Source: CAD feature listing. Evaluate the final solid. Frame: model axes, mm. A direction names the side the tool comes from. Give positions to 0.01 mm unless a question says otherwise; leave off trailing zeros. Loops run counter-clockwise (first coordinate to the right, second up) from the corner with the lowest first, then second, coordinate; pieces in that order, holes last.
from build123d import *

# Parameters (mm, degrees)
BOSS_EXTRUDE1_DEPTH = 25
SKETCH2_R           = 3
CUT_EXTRUDE1_DEPTH  = 11


with BuildPart() as part:
    # Sketch1 → Boss-Extrude1 (new, symmetric)
    with BuildSketch(Plane.XY):
        with BuildLine():
            Line((-24, 23), (24, 23))
            Line((24, 23), (24, -16))
            Line((24, -16), (9.237604307, -16))
            Line((9.237604307, -16), (5, -8.660254038))
            ThreePointArc((5, -8.660254038), (0, 10), (-5, -8.660254038))
            Line((-5, -8.660254038), (-9.237604307, -16))
            Line((-9.237604307, -16), (-24, -16))
            Line((-24, -16), (-24, 23))
        make_face()
    extrude(amount=BOSS_EXTRUDE1_DEPTH, both=True)

    # Sketch2 → Cut-Extrude1 (cut)
    with BuildSketch(Plane(origin=(0, 23, 0), x_dir=(1, 0, 0), z_dir=(0, 1, 0))):
        with Locations(Location((-17.5, 17.5, 0), (0, 0, 270))):
            Circle(SKETCH2_R)
        with Locations(Location((17.5, 17.5, 0), (0, 0, 270))):
            Circle(SKETCH2_R)
        with Locations(Location((17.5, -17.5, 0), (0, 0, 270))):
            Circle(SKETCH2_R)
        with Locations(Location((-17.5, -17.5, 0), (0, 0, 270))):
            Circle(SKETCH2_R)
    extrude(amount=-CUT_EXTRUDE1_DEPTH, mode=Mode.SUBTRACT)


solid = part.part
1) Pull-direction query (X, two-part tool) for faces 4 (the flat face through (-24, 3, 0)), 5 (the flat face through (0, 12, -25)), 6 (the flat face through (-17, 12, -18)); classes: released by +X, released by -X, zero draft, split by the parting line, or undercut.
Checks:
face 4: released by -X
face 5: zero draft
face 6: undercut
2) Contact query for a flat-ended pin moving along its axis: P1, Ø1.8, axis at x = 16.5, z = -18, coming from the +Y side. Output: stop coordinate, or through.
Checks:
P1: stops at y = 12
3) Ray query, probe 1 along X at (y, z) = (14.75, -17.5); probe 2 along X at (y, z) = (0, -12); probe 3 along Z at (x, y) = (-17, 16). Return the intervals inside material, ascending.
Checks:
probe 1: x = -24 to -20.5, -14.5 to 14.5, 20.5 to 24
probe 2: x = -24 to -10, 10 to 24
probe 3: z = -25 to -20.46, -14.54 to 14.54, 20.46 to 25
4) Cut plane D-D (x = 17.5). Return loops of the section in (y, z).
Checks:
outline: (-16, -25) - (23, -25) - (23, -20.5) - (12, -20.5) - (12, -14.5) - (23, -14.5) - (23, 14.5) - (12, 14.5) - (12, 20.5) - (23, 20.5) - (23, 25) - (-16, 25) - close
5) Reachability of faces 1 (the cylindrical face through (-20.43, 17.58, 16.85)), 2 (the flat face through (7.148, -12.382, 0.35)), 3 (the flat face through (24, 4, 0)) from +Z, -Z, +X, -X, +Y, -Y: full face, straight path, thin tool, end or side. Return the list, or none.
Checks:
face 1: +Y
face 2: +Z, -Z, -Y
face 3: +Z, -Z, +X, +Y, -Y
6) Cut plane B-B (y = 13.5). Return loops of the section in (x, z).
Checks:
outline: (-24, -25) - (24, -25) - (24, 25) - (-24, 25) - close; hole circle Ø6 at (-17.5, -17.5); hole circle Ø6 at (-17.5, 17.5); hole circle Ø6 at (17.5, -17.5); hole circle Ø6 at (17.5, 17.5)
7) Cut plane C-C (z = 0). Return loops of the section in (x, y), and give its area (3 significant figures).
Checks:
outline: (-24, -16) - (-9.24, -16) - (-5, -8.66) arc R10 cw (long way) to (5, -8.66) - (9.24, -16) - (24, -16) - (24, 23) - (-24, 23) - close
area: 1,460 mm2
8) Cut plane A-A (y = 8). Return loops of the section in (x, z), and give its area (3 significant figures).
Checks:
outline: (-24, -25) - (-6, -25) - (-6, 25) - (-24, 25) - close; (6, -25) - (24, -25) - (24, 25) - (6, 25) - close
area: 1,800 mm2
